Source: three-view drawing plus pictorial views. Frame: mm from the lowest corner of the part. Coordinates: 2 decimals unless noted, no trailing zeros. Loops run counter-clockwise (first coordinate to the right, second up) from the corner with the lowest first, then second, coordinate; pieces in that order, holes last. Notation, with made-up numbers: (36, -14) - (57, -14) arc R30 ccw to (57, 8) - close; hole circle Ø11 at (17.5, 52). An arc over 180 degrees is marked (long way). Return JSON: item names as keys, results as strings.
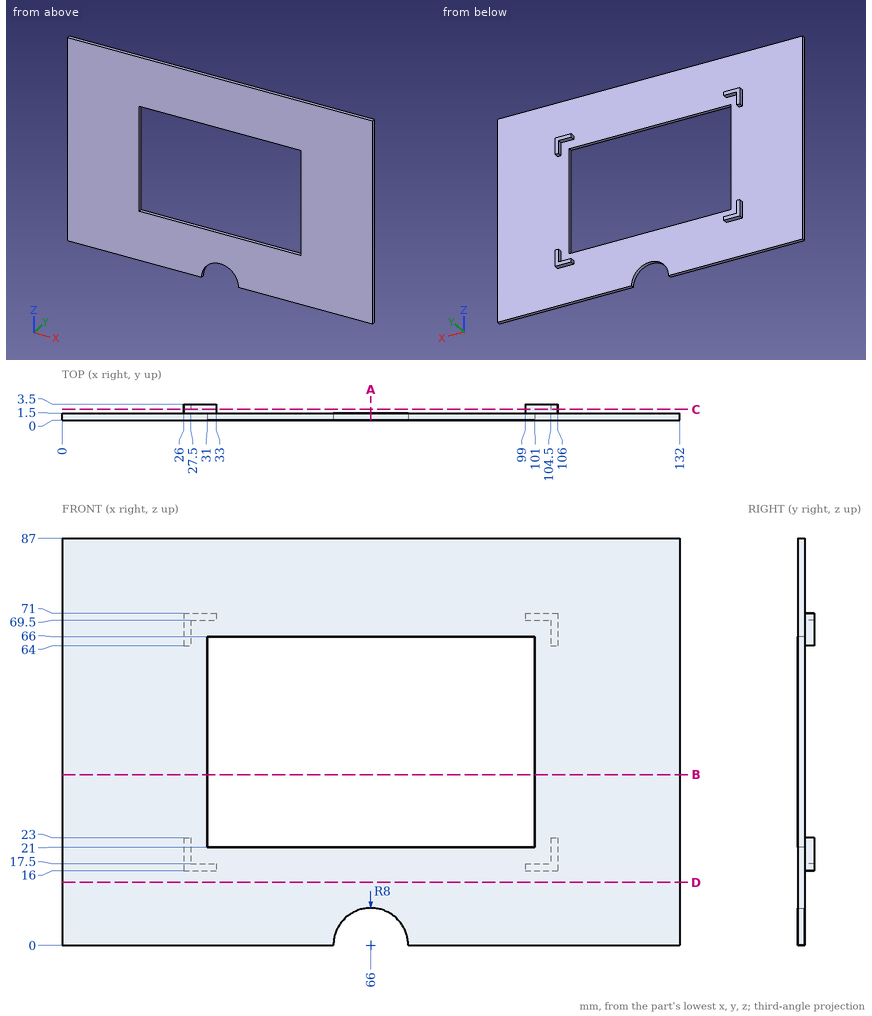
Item 1: First-contact query: pin 1 Ø0.6 at (y, z) = (2.5, 18) entering from +X; pin 2 Ø1 at (x, y) = (31, 2.5) entering from -Z; pin 3 Ø1 at (y, z) = (3, 19.5) entering from -X. Flat tips, straight axial feed; report the tip coordinate or a pass-through.
Worked out:
{"pin 1": "x = 106", "pin 2": "z = 16", "pin 3": "x = 26"}
Item 2: Section query A-A, the plane x = 66. Return loops of the section in (y, z).
Worked out:
{"outline": "(0, 8) - (1.5, 8) - (1.5, 21) - (0, 21) - close; (0, 66) - (1.5, 66) - (1.5, 87) - (0, 87) - close"}
Item 3: Section query D-D, the plane z = 13.5. Return loops of the section in (x, y), and give its area (3 significant figures).
Worked out:
{"outline": "(0, 0) - (132, 0) - (132, 1.5) - (0, 1.5) - close", "area": "198 mm^2"}
Item 4: Ray query, probe 1 along Z at (x, y) = (29, 2.25); probe 2 along X at (y, z) = (0.55, 30); probe 3 along Y at (x, z) = (17, 19). Return the intervals inside material, ascending. Write a range as from..to.
Worked out:
{"probe 1": "16..17.5, 69.5..71", "probe 2": "0..31, 101..132", "probe 3": "0..1.5"}
Item 5: Section query B-B, the plane z = 36.5. Return loops of the section in (x, y).
Worked out:
{"outline": "(0, 0) - (31, 0) - (31, 1.5) - (0, 1.5) - close; (101, 0) - (132, 0) - (132, 1.5) - (101, 1.5) - close"}
Item 6: Section query C-C, the plane y = 2.35. Return loops of the section in (x, z).
Worked out:
{"outline": "(26, 16) - (33, 16) - (33, 17.5) - (27.5, 17.5) - (27.5, 23) - (26, 23) - close; (26, 64) - (27.5, 64) - (27.5, 69.5) - (33, 69.5) - (33, 71) - (26, 71) - close; (99, 16) - (106, 16) - (106, 23) - (104.5, 23) - (104.5, 17.5) - (99, 17.5) - close; (99, 69.5) - (104.5, 69.5) - (104.5, 64) - (106, 64) - (106, 71) - (99, 71) - close"}
